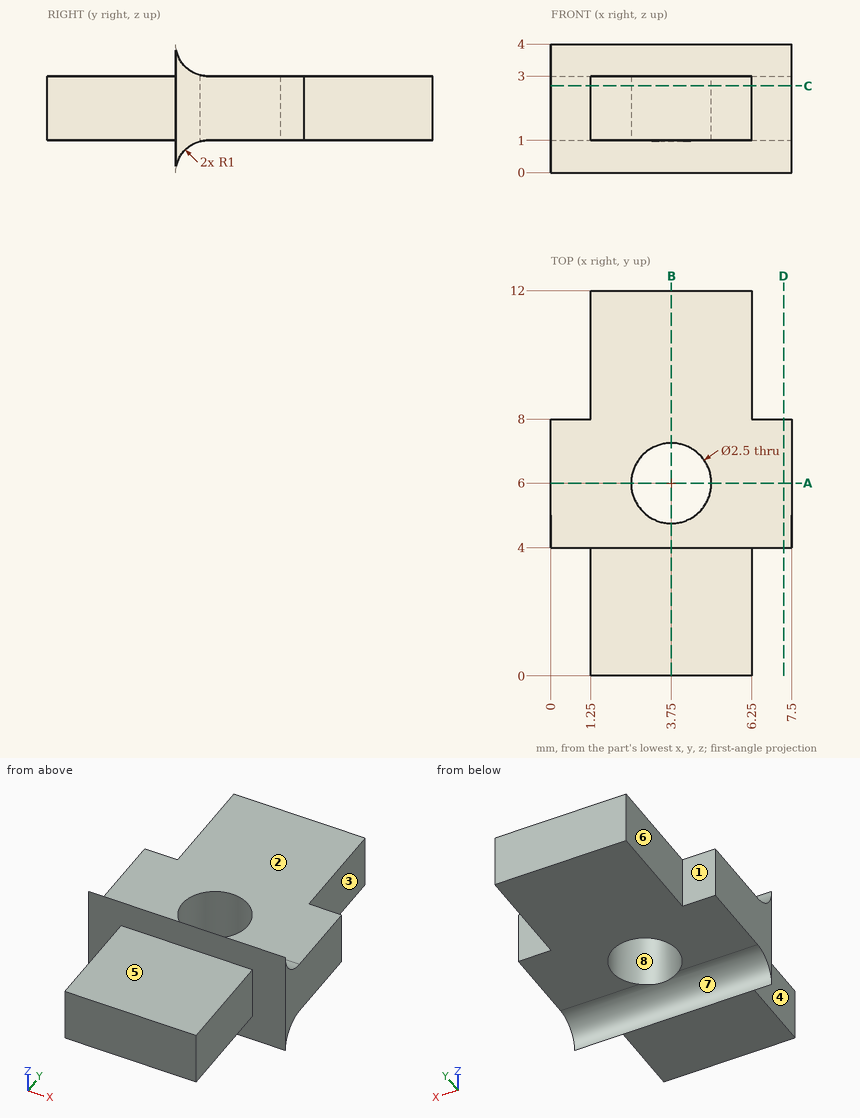
Part print with two shaded views. Sizes in mm from the minimum x, y, z corner. A direction names the side the tool comes from. Round coordinates to 2 decimals unless told otherwise and drop trailing zeros. Write each loop counter-clockwise with the first axis right and the second up, starting at its lowest first coordinate (ties: lowest second). Pieces come first, ordered by that corner, then holes. Notation, with made-up numbers: (45, -1.5) - (101, -1.5) arc R21 cw to (101, 2.5) - close; hole circle Ø5 at (78, 8). An arc over 180 degrees is marked (long way). Use CSV: the item, a comma, the result in double quotes.
Item 1: Tool access for the marked faces 1, 2, 3, 4 and 5: list every direction of +Z, -Z, +X, -X, +Y, -Y with a clear straight run to the whole face (end or side of a thin tool).
Results list:
face 1,"+Z, -Z, -X, +Y"
face 2,"+Z, +X, -X, +Y"
face 3,"+Z, -Z, +X, +Y"
face 4,"+Z, -Z, -X, -Y"
face 5,"+Z, +X, -X, -Y"
Item 2: Slice it at D-D, the plane x = 7.25. Write the cut outline in (y, z), then the cut area to 3 significant figures.
Results list:
outline,"(4, 0) arc R1 cw to (5, 1) - (8, 1) - (8, 3) - (5, 3) arc R1 cw to (4, 4) - close"
area,"8.43 mm²"
Item 3: Slice it at B-B, the plane x = 3.75. Write the cut outline in (y, z).
Results list:
outline,"(0, 1) - (4, 1) - (4, 0) arc R1 cw to (4.75, 0.97) - (4.75, 3.03) arc R1 cw to (4, 4) - (4, 3) - (0, 3) - close; (7.25, 1) - (12, 1) - (12, 3) - (7.25, 3) - close"
Item 4: Flat gauge pins, fed straight in: P1, Ø2, axis at x = 4.5, y = 2, coming from the +Z side; P2, Ø1.6, axis at y = 2.5, z = 2, coming from the +X side; P3, Ø3.5, axis at x = 4.5, y = 10, coming from the -Z side; P4, Ø2, axis at x = 4.5, z = 1.5, coming from the -Y side. Where does each tip first touch, or does it go through?
Results list:
P1,"stops at z = 3"
P2,"stops at x = 6.25"
P3,"stops at z = 1"
P4,"stops at y = 0"
Item 5: Slice it at C-C, the plane z = 2.7. Write the cut outline in (x, y), then the cut area to 3 significant figures.
Results list:
outline,"(0, 4) - (1.25, 4) - (1.25, 0) - (6.25, 0) - (6.25, 4) - (7.5, 4) - (7.5, 8) - (6.25, 8) - (6.25, 12) - (1.25, 12) - (1.25, 8) - (0, 8) - close; hole circle Ø2.5 at (3.75, 6)"
area,"65.1 mm²"
Item 6: Slice it at A-A, the plane y = 6. Write the cut outline in (x, z).
Results list:
outline,"(0, 1) - (2.5, 1) - (2.5, 3) - (0, 3) - close; (5, 1) - (7.5, 1) - (7.5, 3) - (5, 3) - close"
Item 7: Pull direction X, two halves, no side cores. Call the marked faces 6, 7 and 8: pulls with the +X half, pulls with the -X half, needs draft (parallel to the pull), parting line crosses it, or undercut.
Results list:
face 6,"pulls with the -X half"
face 7,"needs draft"
face 8,"undercut"
Item 8: Wall check: L1, parallel to Y at x = 3.75, z = 2.4; L2, parallel to X at y = 6, z = 2.25; L3, parallel to X at y = 3, z = 2.6. Give the ranges that are in metal, low to high.
Results list:
L1,"y = 0 to 4.75, 7.25 to 12"
L2,"x = 0 to 2.5, 5 to 7.5"
L3,"x = 1.25 to 6.25"
